Check sheet for the modelled part. Datum: model origin and axes. Units: mm. A direction names the side the tool comes from. Give positions to 0.01 mm unless a question says otherwise; leave off trailing zeros. Order: outer loops, then holes, each group sorted by start corner. A loop starts at its lowest first (then second) coordinate and runs counter-clockwise, first axis right, second up. Notation, with made-up numbers: (75, 75) -> (108, 75) arc R21 cw to (108, 107) -> close; hole circle Ø11 at (43, 18). An arc over 180 degrees is marked (long way). One line per question, with ' | ' between items.
Autodesk Inventor part; units mm, degrees
ref_plane "YZ Plane" through (0, 0, 0) normal (1, 0, 0) x (0, 1, 0)
ref_plane "XZ Plane" through (0, 0, 0) normal (0, 1, 0) x (-1, 0, 0)
ref_plane "XY Plane" through (0, 0, 0) normal (0, 0, 1) x (1, 0, 0)
sketch "Sketch1" plane through (0, 0, 0) normal (0, 1, 0) x (-1, 0, 0)
  circle A0 centre (12.7, 0) radius 3.175
  line L0 (0, -4.445) -> (0, 4.445)
  point P0 (0, 0)
  dimension "d0" = 12.7
  dimension "d1" = 6.35
revolve "Revolution1" add sketch "Sketch1" angle 180 about axis through (0, 0, -10) along (0, 0, 1)
sketch "Sketch2" plane through (-12.7, 0, 0) normal (0, 1, 0) x (1, 0, 0)
  circle A0 centre (0, 0) radius 3.175
  circle A1 centre (25.4, 0) radius 3.175
  point P0 (12.7, 0)
extrude "Extrusion1" add sketch "Sketch2" along normal blind 6.35
sketch "Sketch3" plane through (-12.7, 6.35, 0) normal (0, 1, 0) x (1, 0, 0)
  circle A0 centre (0, 0) radius 3.175
  circle A1 centre (25.4, 0) radius 3.175
  point P0 (12.7, 0)
extrude "Extrusion2" add sketch "Sketch3" along normal blind 15.875
thread "Thread1"
thread "Thread2"
sketch "Sketch4" plane through (-12.7, 22.225, 0) normal (0, 1, 0) x (1, 0, 0)
  line L0 (-3.2033, 0) -> (28.6033, 0) construction
  line L1 (-3.2033, -3.175) -> (28.6033, -3.175)
  line L2 (28.6033, 3.175) -> (-3.2033, 3.175)
  arc A0 (-3.2033, 3.175) -> (-3.2033, -3.175) centre (-3.2033, 0) ccw
  arc A1 (28.6033, -3.175) -> (28.6033, 3.175) centre (28.6033, 0) ccw
  point P0 (12.7, 0)
extrude "Extrusion3" cut sketch "Sketch4" against normal blind 5
properties part number "19mm ID UBOLT" material "Stainless Steel, 440C"
Q1. Mould release check, pull along X, two halves, no side actions. Record for faces 1 (the face through (-9.67, 8.49, 0.95)), 2 (the face through (13, 17.225, 0)): pulls with the +X half, pulls with the -X half, needs draft (parallel to the pull), parting line crosses it, or undercut.
Result sheet:
face 1: undercut | face 2: needs draft
Q2. Access from +Z, -Z, +X, -X, +Y, -Y to the whole of each face (thin tool, end or side, straight path). Record for faces 3 (the face through (-13, 17.225, 0)), 4 (the face through (9.53, 8.49, 0.14)).
Result sheet:
face 3: +Z, -Z, +X, -X, +Y | face 4: +Y
Q3. Section check C-C (z = 2.5). Enter the section's corners in (x, y) (3 decimals), and give its area (3 significant figures).
Result sheet:
outline: (-14.657, 0) arc R14.657 ccw to (14.657, 0) -> (14.657, 17.225) -> (10.743, 17.225) -> (10.743, 0) arc R10.743 cw to (-10.743, 0) -> (-10.743, 17.225) -> (-14.657, 17.225) -> close | area: 291 mm2
Q4. Section check B-B (z = 0). Enter the section's corners in (x, y) (3 decimals).
Result sheet:
outline: (-15.875, 0) arc R15.875 ccw to (15.875, 0) -> (15.875, 17.225) -> (9.525, 17.225) -> (9.525, 0) arc R9.525 cw to (-9.525, 0) -> (-9.525, 17.225) -> (-15.875, 17.225) -> close
Q5. Section check A-A (y = 14.5). Enter the section's corners in (x, z) (3 decimals).
Result sheet:
outline: circle Ø6.35 at (-12.7, 0); circle Ø6.35 at (12.7, 0)
Q6. Depth check by flat-ended pin: pin 1 Ø2 at (y, z) = (4, -2.5) entering from -X; pin 2 Ø3 at (x, z) = (5, 1) entering from -Y. Enter the tip coordinate at first touch or a pass-through.
Result sheet:
pin 1: stops at x = -15.5 | pin 2: stops at y = -15.43
Q7. Thickness scan on line 1 (X direction, y = 16.5, z = -2.25); line 2 (X direction, y = 3, z = -2.5); line 3 (Z direction, x = 11.5, y = -5). Record the ranges inside material, lowest first.
Result sheet:
line 1: x = -14.94 to -10.46, 10.46 to 14.94 | line 2: x = -14.66 to -10.74, 10.74 to 14.66 | line 3: z = -3.17 to 3.17
